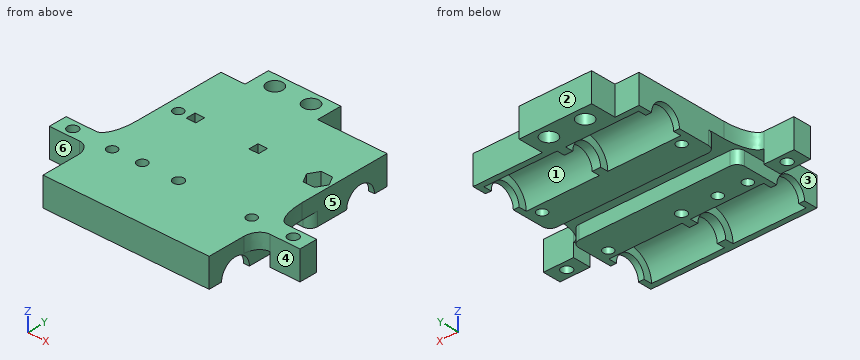
from build123d import *

# Parameters (mm, degrees)
SZKIC8_W                        = 55
SZKIC8_H                        = 64
DODANIE_WYCI_GNI_CIE3_DEPTH     = 9.5
WYTNIJ_WYCI_GNI_CIE2_START      = -1.9
SZKIC9_R                        = 7.6
WYTNIJ_WYCI_GNI_CIE2_DEPTH      = 24.2
WYTNIJ_WYCI_GNI_CIE3_START      = -1.9
SZKIC10_R                       = 7.65
WYTNIJ_WYCI_GNI_CIE3_DEPTH      = 24.2
WYTNIJ_WYCI_GNI_CIE4_DEPTH      = 71.763691255
WYTNIJ_WYCI_GNI_CIE4_DEPTH_BACK = 71.763691255
SZKIC11_R                       = 5
WYTNIJ_WYCI_GNI_CIE25_REACH     = 54.333
SZKIC42_R                       = 1.65
SZKIC43_W                       = 24
SZKIC43_H                       = 8.4
DODANIE_WYCI_GNI_CIE4_DEPTH     = 9.5
WYTNIJ_WYCI_GNI_CIE26_REACH     = 61.499
SZKIC44_R                       = 2.65
SZKIC45_W                       = 3.2
SZKIC45_H                       = 3.2
WYTNIJ_WYCI_GNI_CIE27_DEPTH     = 3.4
SZKIC46_R                       = 1.7
SZKIC46_R_2                     = 1.75
WYTNIJ_WYCI_GNI_CIE28_DEPTH     = 60.498823518
WYTNIJ_WYCI_GNI_CIE29_DEPTH     = 4.5
SZKIC49_W                       = 10
SZKIC49_H                       = 6
DODANIE_WYCI_GNI_CIE5_DEPTH     = 4.5
DODANIE_WYCI_GNI_CIE5_2_DEPTH   = 4.5
SZKIC50_W                       = 14
SZKIC50_H                       = 6
DODANIE_WYCI_GNI_CIE6_DEPTH     = 5
WYTNIJ_WYCI_GNI_CIE31_REACH     = 69.128
SZKIC51_R                       = 1.75
ZAOKR_GLENIE2_SIZE              = 10
ZAOKR_GLENIE2_SIZE_2            = 4
ZAOKR_GLENIE3_SIZE              = 4
ZAOKR_GLENIE3_SIZE_2            = 5
SZKIC52_W                       = 55
SZKIC52_H                       = 8
WYTNIJ_WYCI_GNI_CIE32_DEPTH     = 4.5
ZAOKR_GLENIE4_R                 = 2.5


with BuildPart() as part:
    # Szkic8 → Dodanie-wyci_gni_cie3 (new body)
    with BuildSketch(Plane.XY):
        with Locations((0, 11.5)):
            Rectangle(SZKIC8_W, SZKIC8_H)
    extrude(amount=DODANIE_WYCI_GNI_CIE3_DEPTH)

    # Szkic9 → Wytnij-wyci_gni_cie2 (cut)
    with BuildSketch(Plane(origin=(27.5, 0, 0), x_dir=(0, 0, -1), z_dir=(1, 0, 0)).offset(WYTNIJ_WYCI_GNI_CIE2_START)):
        with Locations((0, 34)):
            Circle(SZKIC9_R)
    wytnij_wyci_gni_cie2 = extrude(amount=-WYTNIJ_WYCI_GNI_CIE2_DEPTH, mode=Mode.SUBTRACT)

    # Szkic10 → Wytnij-wyci_gni_cie3 (cut)
    with BuildSketch(Plane(origin=(27.5, 0, 0), x_dir=(0, 0, -1), z_dir=(1, 0, 0)).offset(WYTNIJ_WYCI_GNI_CIE3_START)):
        with Locations((0, -11)):
            Circle(SZKIC10_R)
    wytnij_wyci_gni_cie3 = extrude(amount=-WYTNIJ_WYCI_GNI_CIE3_DEPTH, mode=Mode.SUBTRACT)

    # Lustro4: Wytnij-wyci_gni_cie2, Wytnij-wyci_gni_cie3 across plane
    add(wytnij_wyci_gni_cie2.mirror(Plane(origin=(0, 0, 0), x_dir=(0, 0, 1), z_dir=(1, 0, 0))), mode=Mode.SUBTRACT)
    add(wytnij_wyci_gni_cie3.mirror(Plane(origin=(0, 0, 0), x_dir=(0, 0, 1), z_dir=(1, 0, 0))), mode=Mode.SUBTRACT)

    # Szkic11 → Wytnij-wyci_gni_cie4 (cut, two sides: drawn at the far end of the back side and taken through both)
    with BuildSketch(Plane(origin=(27.5, 0, 0), x_dir=(0, 0, -1), z_dir=(1, 0, 0)).offset(-WYTNIJ_WYCI_GNI_CIE4_DEPTH_BACK)):
        with Locations((0, 34)):
            Circle(SZKIC11_R)
        with Locations((0, -11)):
            Circle(SZKIC11_R)
    extrude(amount=WYTNIJ_WYCI_GNI_CIE4_DEPTH + WYTNIJ_WYCI_GNI_CIE4_DEPTH_BACK, mode=Mode.SUBTRACT)

    # Szkic42 → Wytnij-wyci_gni_cie25 (cut, up to next)
    with BuildSketch(Plane(origin=(0, 0, 0), x_dir=(-1, 0, 0), z_dir=(0, 0, -1)), mode=Mode.PRIVATE) as wytnij_wyci_gni_cie25_sk1:
        with Locations((23.1, 23.4)):
            Circle(SZKIC42_R)
    wytnij_wyci_gni_cie25_tool1 = extrude(wytnij_wyci_gni_cie25_sk1.sketch, amount=-WYTNIJ_WYCI_GNI_CIE25_REACH, mode=Mode.PRIVATE) & part.part
    # Szkic42 → Wytnij-wyci_gni_cie25 (cut, up to next)
    with BuildSketch(Plane(origin=(0, 0, 0), x_dir=(-1, 0, 0), z_dir=(0, 0, -1)), mode=Mode.PRIVATE) as wytnij_wyci_gni_cie25_sk2:
        with Locations((23.1, -0.4)):
            Circle(SZKIC42_R)
    wytnij_wyci_gni_cie25_tool2 = extrude(wytnij_wyci_gni_cie25_sk2.sketch, amount=-WYTNIJ_WYCI_GNI_CIE25_REACH, mode=Mode.PRIVATE) & part.part
    # Szkic42 → Wytnij-wyci_gni_cie25 (cut, up to next)
    with BuildSketch(Plane(origin=(0, 0, 0), x_dir=(-1, 0, 0), z_dir=(0, 0, -1)), mode=Mode.PRIVATE) as wytnij_wyci_gni_cie25_sk3:
        with Locations((-23.1, -0.4)):
            Circle(SZKIC42_R)
    wytnij_wyci_gni_cie25_tool3 = extrude(wytnij_wyci_gni_cie25_sk3.sketch, amount=-WYTNIJ_WYCI_GNI_CIE25_REACH, mode=Mode.PRIVATE) & part.part
    # Szkic42 → Wytnij-wyci_gni_cie25 (cut, up to next)
    with BuildSketch(Plane(origin=(0, 0, 0), x_dir=(-1, 0, 0), z_dir=(0, 0, -1)), mode=Mode.PRIVATE) as wytnij_wyci_gni_cie25_sk4:
        with Locations((-23.1, 23.4)):
            Circle(SZKIC42_R)
    wytnij_wyci_gni_cie25_tool4 = extrude(wytnij_wyci_gni_cie25_sk4.sketch, amount=-WYTNIJ_WYCI_GNI_CIE25_REACH, mode=Mode.PRIVATE) & part.part
    add(wytnij_wyci_gni_cie25_tool1.solids().sort_by_distance((-23.1, 23.4, 0))[0], mode=Mode.SUBTRACT)
    add(wytnij_wyci_gni_cie25_tool2.solids().sort_by_distance((-23.1, -0.4, 0))[0], mode=Mode.SUBTRACT)
    add(wytnij_wyci_gni_cie25_tool3.solids().sort_by_distance((23.1, -0.4, 0))[0], mode=Mode.SUBTRACT)
    add(wytnij_wyci_gni_cie25_tool4.solids().sort_by_distance((23.1, 23.4, 0))[0], mode=Mode.SUBTRACT)

    # Szkic43 → Dodanie-wyci_gni_cie4 (add)
    with BuildSketch(Plane.XY.offset(9.5)):
        with Locations((-7.5, 47.7)):
            Rectangle(SZKIC43_W, SZKIC43_H)
    extrude(amount=-DODANIE_WYCI_GNI_CIE4_DEPTH)

    # Szkic44 → Wytnij-wyci_gni_cie26 (cut, up to next)
    with BuildSketch(Plane.XY.offset(9.5), mode=Mode.PRIVATE) as wytnij_wyci_gni_cie26_sk1:
        with Locations((-13.5, 47.7)):
            Circle(SZKIC44_R)
    wytnij_wyci_gni_cie26_tool1 = extrude(wytnij_wyci_gni_cie26_sk1.sketch, amount=-WYTNIJ_WYCI_GNI_CIE26_REACH, mode=Mode.PRIVATE) & part.part
    # Szkic44 → Wytnij-wyci_gni_cie26 (cut, up to next)
    with BuildSketch(Plane.XY.offset(9.5), mode=Mode.PRIVATE) as wytnij_wyci_gni_cie26_sk2:
        with Locations((-1.5, 47.7)):
            Circle(SZKIC44_R)
    wytnij_wyci_gni_cie26_tool2 = extrude(wytnij_wyci_gni_cie26_sk2.sketch, amount=-WYTNIJ_WYCI_GNI_CIE26_REACH, mode=Mode.PRIVATE) & part.part
    add(wytnij_wyci_gni_cie26_tool1.solids().sort_by_distance((-13.5, 47.7, 9.5))[0], mode=Mode.SUBTRACT)
    add(wytnij_wyci_gni_cie26_tool2.solids().sort_by_distance((-1.5, 47.7, 9.5))[0], mode=Mode.SUBTRACT)

    # Szkic45 → Wytnij-wyci_gni_cie27 (cut)
    with BuildSketch(Plane.XY.offset(9.5)):
        with Locations((-17.9, 23.9)):
            Rectangle(SZKIC45_W, SZKIC45_H)
        with Locations((2.9, 23.9)):
            Rectangle(SZKIC45_W, SZKIC45_H)
    extrude(amount=-WYTNIJ_WYCI_GNI_CIE27_DEPTH, mode=Mode.SUBTRACT)

    # Szkic46 → Wytnij-wyci_gni_cie28 (cut, through all)
    with BuildSketch(Plane.XY.offset(9.5)):
        with Locations((-13.5, 0)):
            Circle(SZKIC46_R)
        with Locations((-1.5, 0)):
            Circle(SZKIC46_R_2)
    extrude(amount=-WYTNIJ_WYCI_GNI_CIE28_DEPTH, mode=Mode.SUBTRACT)

    # Szkic47 → Wytnij-wyci_gni_cie29 (cut)
    with BuildSketch(Plane.XY.offset(9.5)):
        Polygon((21.223611625, 20.15), (24.976388375, 20.15), (26.85277675, 23.4), (24.976388375, 26.65), (21.223611625, 26.65), (19.34722325, 23.4), align=None)
    extrude(amount=-WYTNIJ_WYCI_GNI_CIE29_DEPTH, mode=Mode.SUBTRACT)



with BuildPart() as body_2:
    # Szkic49 → Dodanie-wyci_gni_cie5 (new body)
    with BuildSketch(Plane(origin=(0, 0, 0), x_dir=(-1, 0, 0), z_dir=(0, 0, -1))):
        with Locations((36.5, 0)):
            Rectangle(SZKIC49_W, SZKIC49_H)
    extrude(amount=-DODANIE_WYCI_GNI_CIE5_DEPTH)


with BuildPart() as body_3:
    # Szkic49 → Dodanie-wyci_gni_cie5 2 (new body)
    with BuildSketch(Plane(origin=(0, 0, 0), x_dir=(-1, 0, 0), z_dir=(0, 0, -1))):
        with Locations((-36.5, 0)):
            Rectangle(SZKIC49_W, SZKIC49_H)
    extrude(amount=-DODANIE_WYCI_GNI_CIE5_2_DEPTH)


with BuildPart() as part_1:
    add(part.part)

    add(body_2.part)  # Dodanie-wyci_gni_cie6 merges body 2

    add(body_3.part)  # Dodanie-wyci_gni_cie6 merges body 3
    # Szkic50 → Dodanie-wyci_gni_cie6 (add)
    with BuildSketch(Plane.XY.offset(4.5)):
        with Locations((-34.5, 0)):
            Rectangle(SZKIC50_W, SZKIC50_H)
        with Locations((34.5, 0)):
            Rectangle(SZKIC50_W, SZKIC50_H)
    extrude(amount=DODANIE_WYCI_GNI_CIE6_DEPTH)

    # Szkic51 → Wytnij-wyci_gni_cie31 (cut, up to next)
    with BuildSketch(Plane(origin=(0, 0, 0), x_dir=(-1, 0, 0), z_dir=(0, 0, -1)), mode=Mode.PRIVATE) as wytnij_wyci_gni_cie31_sk1:
        with Locations((36.5, 0)):
            Circle(SZKIC51_R)
    wytnij_wyci_gni_cie31_tool1 = extrude(wytnij_wyci_gni_cie31_sk1.sketch, amount=-WYTNIJ_WYCI_GNI_CIE31_REACH, mode=Mode.PRIVATE) & part_1.part
    # Szkic51 → Wytnij-wyci_gni_cie31 (cut, up to next)
    with BuildSketch(Plane(origin=(0, 0, 0), x_dir=(-1, 0, 0), z_dir=(0, 0, -1)), mode=Mode.PRIVATE) as wytnij_wyci_gni_cie31_sk2:
        with Locations(Location((-36.5, 0, 0), (0, 0, 180))):
            Circle(SZKIC51_R)
    wytnij_wyci_gni_cie31_tool2 = extrude(wytnij_wyci_gni_cie31_sk2.sketch, amount=-WYTNIJ_WYCI_GNI_CIE31_REACH, mode=Mode.PRIVATE) & part_1.part
    add(wytnij_wyci_gni_cie31_tool1.solids().sort_by_distance((-36.5, 0, 0))[0], mode=Mode.SUBTRACT)
    add(wytnij_wyci_gni_cie31_tool2.solids().sort_by_distance((36.5, 0, 0))[0], mode=Mode.SUBTRACT)

    # Zaokr_glenie2
    # an asymmetric fillet: 10, 4 mm, written as the material it adds along each edge
    with BuildSketch(Plane(origin=(-27.5, 3, 4.5), x_dir=(0, 1, 0), z_dir=(0, 0, 1))) as zaokr_glenie2_piece_1:
        with BuildLine():
            Bezier((ZAOKR_GLENIE2_SIZE, 0), (0, 0), (0, ZAOKR_GLENIE2_SIZE_2), weights=[1, 0.707106781, 1])
            Line((0, ZAOKR_GLENIE2_SIZE_2), (0, 0))
            Line((0, 0), (ZAOKR_GLENIE2_SIZE, 0))
        make_face()
    extrude(amount=5)
    with BuildSketch(Plane(origin=(27.5, 3, 4.5), x_dir=(0, 1, 0), z_dir=(0, 0, 1))) as zaokr_glenie2_piece_2:
        with BuildLine():
            Bezier((ZAOKR_GLENIE2_SIZE, 0), (0, 0), (0, -ZAOKR_GLENIE2_SIZE_2), weights=[1, 0.707106781, 1])
            Line((0, -ZAOKR_GLENIE2_SIZE_2), (0, 0))
            Line((0, 0), (ZAOKR_GLENIE2_SIZE, 0))
        make_face()
    extrude(amount=5)

    # Zaokr_glenie3
    # an asymmetric fillet: 5, 4 mm, written as the material it adds along each edge
    with BuildSketch(Plane(origin=(-27.5, -3, 4.5), x_dir=(-1, 0, 0), z_dir=(0, 0, 1))) as zaokr_glenie3_piece_1:
        with BuildLine():
            Bezier((ZAOKR_GLENIE3_SIZE, 0), (0, 0), (0, ZAOKR_GLENIE3_SIZE_2), weights=[1, 0.707106781, 1])
            Line((0, ZAOKR_GLENIE3_SIZE_2), (0, 0))
            Line((0, 0), (ZAOKR_GLENIE3_SIZE, 0))
        make_face()
    extrude(amount=5)
    with BuildSketch(Plane(origin=(27.5, -3, 4.5), x_dir=(1, 0, 0), z_dir=(0, 0, 1))) as zaokr_glenie3_piece_2:
        with BuildLine():
            Bezier((ZAOKR_GLENIE3_SIZE, 0), (0, 0), (0, -ZAOKR_GLENIE3_SIZE_2), weights=[1, 0.707106781, 1])
            Line((0, -ZAOKR_GLENIE3_SIZE_2), (0, 0))
            Line((0, 0), (ZAOKR_GLENIE3_SIZE, 0))
        make_face()
    extrude(amount=5)

    # Szkic52 → Wytnij-wyci_gni_cie32 (cut)
    with BuildSketch(Plane(origin=(0, 0, 0), x_dir=(-1, 0, 0), z_dir=(0, 0, -1))):
        with Locations((0, 12)):
            Rectangle(SZKIC52_W, SZKIC52_H)
    extrude(amount=-WYTNIJ_WYCI_GNI_CIE32_DEPTH, mode=Mode.SUBTRACT)

    # Zaokr_glenie4
    zaokr_glenie4_edges = [part_1.edges().sort_by_distance(p)[0] for p in [
        (27.5, 8, 2.25),
        (27.5, 16, 2.25),
        (-27.5, 8, 2.25),
        (-27.5, 16, 2.25),
    ]]
    fillet(zaokr_glenie4_edges, radius=ZAOKR_GLENIE4_R)


solid = part_1.part
Verification items for the finished model (mm, model axes). Face numbers are marked on the shaded views. A direction names the side the tool comes from. Round coordinates to 2 decimals unless told otherwise and drop trailing zeros. Loops run counter-clockwise (first coordinate to the right, second up) from the corner with the lowest first, then second, coordinate; pieces in that order, holes last. Notation, with made-up numbers: (-24.5, -1.75) - (33.5, -1.75) arc R7 ccw to (33.5, 5.25) - close; hole circle Ø8 at (87.25, 34). An arc over 180 degrees is marked (long way). Answer in a Markdown table with one row per item. Add a question column.
Q1. Tool access check on the marked faces 4, 5 and 6. Record the directions out of +Z, -Z, +X, -X, +Y, -Y that give a thin tool (end or side, any length) a straight path to the whole face; none if there is none.
Q2. Gauge pin test, flat ends, axial feed: pin 1 (2 mm diameter, centred on y = 22.5, z = 7.5, fed in from +X); pin 2 (21 mm diameter, centred on x = 6, y = 1.5, fed in from -Z); pin 3 (4 mm diameter, centred on y = -10, z = 3, fed in from -X); pin 4 (3 mm diameter, centred on x = -35, z = 5.5, fed in from -Y). Record the tip position at first contact, or that the pin passes through.
Q3. Material ranges on line 1 (X direction, y = 35.5, z = 5.5); line 2 (Y direction, x = -13.5, z = 0.5); line 3 (X direction, y = 22, z = 3.5), recorded low to high.
Q4. Section check B-B on y = 47.7. Enter the section's corners in (x, z), plus the area to 3 significant figures.
Q5. Section check A-A on x = 23.1. Enter the section's corners in (y, z), plus the area to 3 significant figures.
Q6. Release check for a two-part mould opening along Y. For the marked faces 1, 2 and 3 record: pulls with the +Y half, pulls with the -Y half, needs draft (parallel to the pull), parting line crosses it, or undercut.
Q7. Section check C-C on y = -11. Enter the section's corners in (x, z), plus the area to 3 significant figures.
Found:
| question | item | result |
|---|---|---|
| 1 | face 4 | +Z, -Z, +X, -Y |
| 1 | face 5 | +Z, -Z, +X, +Y |
| 1 | face 6 | +Z, -Z, -X, -Y |
| 2 | pin 1 | stops at x = 27.5 |
| 2 | pin 2 | stops at z = 0 |
| 2 | pin 3 | stops at x = -27.5 |
| 2 | pin 4 | stops at y = -3 |
| 3 | line 1 | x = -27.5 to -25.6, -1.4 to 1.4, 25.6 to 27.5 |
| 3 | line 2 | y = -20.5 to -18.63, -3.37 to -1.7, 1.7 to 8, 16 to 26.42, 41.58 to 45.05, 50.35 to 51.9 |
| 3 | line 3 | x = -27.5 to -23.97, -22.23 to 22.23, 23.97 to 27.5 |
| 4 | outline | (-19.5, 0) - (-16.15, 0) - (-16.15, 9.5) - (-19.5, 9.5) - close; (-10.85, 0) - (-4.15, 0) - (-4.15, 9.5) - (-10.85, 9.5) - close; (1.15, 0) - (4.5, 0) - (4.5, 9.5) - (1.15, 9.5) - close |
| 4 | area | 127 mm² |
| 5 | outline | (-20.5, 0) - (-18.65, 0) arc R7.65 cw to (-3.35, 0) - (-2.05, 0) - (-2.05, 9.5) - (-20.5, 9.5) - close; (1.25, 0) - (8, 0) - (8, 4.5) - (16, 4.5) - (16, 0) - (21.75, 0) - (21.75, 5) - (20.15, 5) - (20.15, 9.5) - (1.25, 9.5) - close; (25.05, 0) - (26.4, 0) arc R7.6 cw to (41.6, 0) - (43.5, 0) - (43.5, 9.5) - (26.65, 9.5) - (26.65, 5) - (25.05, 5) - close |
| 5 | area | 312 mm² |
| 6 | face 1 | undercut |
| 6 | face 2 | pulls with the +Y half |
| 6 | face 3 | needs draft |
| 7 | outline | (-27.5, 5) - (-25.6, 5) - (-25.6, 7.65) - (-1.4, 7.65) - (-1.4, 5) - (1.4, 5) - (1.4, 7.65) - (25.6, 7.65) - (25.6, 5) - (27.5, 5) - (27.5, 9.5) - (-27.5, 9.5) - close |
| 7 | area | 119 mm² |
